The listing builds one solid part. Answer for the finished solid, in the listing's coordinates (mm). Face numbers are marked on the shaded views. Coordinates: 2 decimals unless noted, no trailing zeros. Order: outer loops, then holes, each group sorted by start corner. A loop starts at its lowest first (then second) coordinate and runs counter-clockwise, first axis right, second up. Notation, with made-up numbers: (-12.5, 17.25) -> (12.5, 17.25) arc R30 ccw to (12.5, 56.25) -> close; hole circle Ø6 at (66, 76). An arc over 180 degrees is marked (long way). Put each result on its own line as item: value. Start each with the question number.
```python
from build123d import *

# Parameters (mm, degrees)
F2_R     = 30
F3_DEPTH = 15.001


with BuildPart() as f1:
    # F0 (on Front) → F1 (revolve)
    with BuildSketch(Plane.XZ):
        Polygon((-5.5, -4), (-4.9, 0), (-4.9, 8), (-4.05, 11), (-4.9, 11), (-30, 11), (-30, -4), align=None)
    revolve(axis=Axis((0, 0, 7.003904), (0, 0, 1)))

    # F2 (on face) → F3 (cut, through all)
    with BuildSketch(Plane.XY.offset(11)):
        Circle(F2_R)
        Polygon((0, 9.179869), (7.95, 4.589935), (7.95, -4.589935), (0, -9.179869), (-7.95, -4.589935), (-7.95, 4.589935), align=None, mode=Mode.SUBTRACT)
    extrude(amount=-F3_DEPTH, mode=Mode.SUBTRACT)


solid = f1.part
```
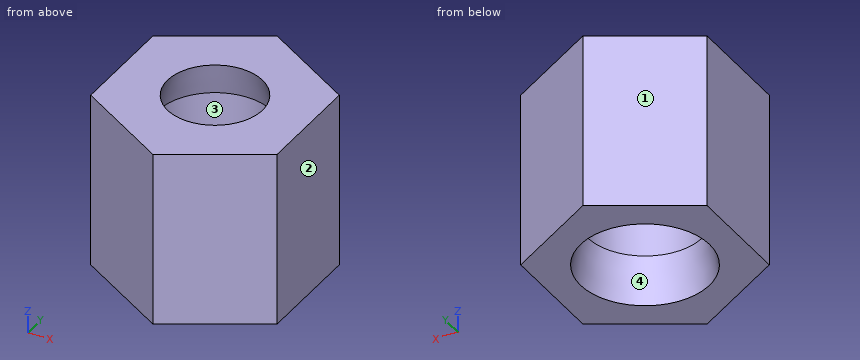
(1) For a pull along Y with two mould halves and no side action, classify the marked faces 1, 2, 3 and 4 as released by +Y, released by -Y, zero draft, split by the parting line, or undercut.
(2) This flat-tipped pin is pushed along its axis until it touches: P1, Ø1.5, axis at x = 3, z = 0.5, coming from the -Y side. Where does it stop, or does it pass through?
(3) The part is cut by section B-B on z = 0.25. Determine the outline of the cut face in (x, y), plus the area to 3 significant figures.
(4) Find the intervals of material crossed by L1, parallel to X at y = 0, z = 2.5; L2, parallel to Y at x = 0.5, z = -0.5; L3, parallel to Y at x = 0.5, z = -1.75, in increasing order.
(5) The part is cut by section D-D on x = -6.25. Determine the outline of the cut face in (y, z), plus the area to 3 significant figures.
(6) The part is cut by section A-A on y = 0. Determine the outline of the cut face in (x, z), plus the area to 4 significant figures.
(7) The part is cut by section C-C on z = 9. Determine the outline of the cut face in (x, y).
Worked out:
1. face 1: released by +Y
1. face 2: zero draft
1. face 3: undercut
1. face 4: undercut
2. P1: y = -7.88
3. outline: (-7.95, -4.59) -> (0, -9.18) -> (7.95, -4.59) -> (7.95, 4.59) -> (0, 9.18) -> (-7.95, 4.59) -> close; hole circle Ø9.8 at (0, 0)
3. area: 144 mm2
4. L1: -7.95 to -4.9, 4.9 to 7.95
4. L2: -8.89 to -4.95, 4.95 to 8.89
4. L3: -8.89 to -5.14, 5.14 to 8.89
5. outline: (-5.57, -4) -> (5.57, -4) -> (5.57, 11) -> (-5.57, 11) -> close
5. area: 167 mm2
6. outline: (-7.95, -4) -> (-5.5, -4) -> (-4.9, 0) -> (-4.9, 8) -> (-4.05, 11) -> (-7.95, 11) -> close; (4.05, 11) -> (4.9, 8) -> (4.9, 0) -> (5.5, -4) -> (7.95, -4) -> (7.95, 11) -> close
6. area: 91.65 mm2
7. outline: (-7.95, -4.59) -> (0, -9.18) -> (7.95, -4.59) -> (7.95, 4.59) -> (0, 9.18) -> (-7.95, 4.59) -> close; hole circle Ø9.23 at (0, 0)
